```python
from build123d import *

# Parameters (mm, degrees)
SKETCH1_R           = 20.5
BOSS_EXTRUDE1_DEPTH = 2
SKETCH2_R           = 2.675
CUT_EXTRUDE1_DEPTH  = 2
BOSS_EXTRUDE2_START = 0.4
SKETCH3_R           = 3.425
SKETCH3_R_2         = 2.675
BOSS_EXTRUDE2_DEPTH = 0.4
SKETCH4_R           = 2
CUT_EXTRUDE2_DEPTH  = 2


with BuildPart() as part:
    # Sketch1 → Boss-Extrude1 (new body)
    with BuildSketch(Plane(origin=(0, 0, 0), x_dir=(1, 0, 0), z_dir=(0, 1, 0))):
        with Locations(Location((0, 0, 0), (0, 0, 270))):
            Circle(SKETCH1_R)
    extrude(amount=BOSS_EXTRUDE1_DEPTH)

    # Sketch2 → Cut-Extrude1 (cut)
    with BuildSketch(Plane(origin=(0, 2, 0), x_dir=(1, 0, 0), z_dir=(0, 1, 0))):
        with Locations(Location((0, 0, 0), (0, 0, 270))):
            Circle(SKETCH2_R)
    extrude(amount=-CUT_EXTRUDE1_DEPTH, mode=Mode.SUBTRACT)

    # Sketch3 → Boss-Extrude2 (add)
    with BuildSketch(Plane(origin=(0, 2, 0), x_dir=(1, 0, 0), z_dir=(0, 1, 0)).offset(BOSS_EXTRUDE2_START)):
        with Locations(Location((0, 0, 0), (0, 0, 270))):
            Circle(SKETCH3_R)
        with Locations(Location((0, 0, 0), (0, 0, 270))):
            Circle(SKETCH3_R_2, mode=Mode.SUBTRACT)
    extrude(amount=-BOSS_EXTRUDE2_DEPTH)

    # Sketch4 → Cut-Extrude2 (cut)
    with BuildSketch(Plane(origin=(0, 2, 0), x_dir=(1, 0, 0), z_dir=(0, 1, 0))):
        with Locations(Location((0, 16.68859089, 0), (0, 0, 270))):
            Circle(SKETCH4_R)
    extrude(amount=-CUT_EXTRUDE2_DEPTH, mode=Mode.SUBTRACT)


solid = part.part
```
Design review of the part built by this model. Coordinates are the model's own, in mm. A direction names the side the tool comes from. Give positions to 0.01 mm unless a question says otherwise; leave off trailing zeros. Write each loop counter-clockwise with the first axis right and the second up, starting at its lowest first coordinate (ties: lowest second). Pieces come first, ordered by that corner, then holes. Notation, with made-up numbers: (-40, 48) - (19, 48) arc R23 ccw to (19, 75) - close; hole circle Ø7 at (48.25, 59.25). An arc over 180 degrees is marked (long way). Return JSON: item names as keys, results as strings. Group by question number.
(1) Machinability: for faces 1 (the cylindrical face through (1.029, 2.203, 3.267)), 2 (the cylindrical face through (-2.61, 1.22, -0.58)), which of the approach directions +Z, -Z, +X, -X, +Y, -Y give a long, thin tool a straight path to every point of the face, cutting with its end or side? Answer none if there is none.
(2) Mouldability with a two-part tool opening along X and no side actions: class faces 3 (the cylindrical face through (-20.013, 0.986, -4.444)), 4 (the cylindrical face through (-0.766, 1.014, -14.841)), 5 (the flat face through (0, 0, 4)) as +X half, -X half, draft (parallel to the pull), parting line (faces both ways), or undercut.
(3) We need section C-C, the plane y = 1.5. Give the boundary of the cut face in (x, z) (3 decimals), then the cut area to 3 significant figures.
(4) We need section D-D, the plane x = 4.5. Give the boundary of the cut face in (y, z), then the cut area to 3 significant figures.
(5) We need section B-B, the plane z = 0. Give the boundary of the cut face in (x, y) (3 decimals).
(6) To check wall thickness, follow probe 1 along X at (y, z) = (0.8, 0) (3 decimals); probe 2 along Z at (x, y) = (1.5, 0.2); probe 3 along Y at (x, z) = (12.5, -4). State the ranges of each line that lie inside material, in increasing order.
(7) We need section A-A, the plane x = 0. Give the boundary of the cut face in (y, z) (3 decimals), then the cut area to 3 significant figures.
Reported:
{
 "1": {"face 1": "+Y", "face 2": "+Y, -Y"},
 "2": {"face 3": "parting line", "face 4": "undercut", "face 5": "draft"},
 "3": {"outline": "circle Ø41 at (0, 0); hole circle Ø5.35 at (0, 0); hole circle Ø4 at (0, -16.689)", "area": "1,290 mm2"},
 "4": {"outline": "(0, -20) - (2, -20) - (2, 20) - (0, 20) - close", "area": "80.0 mm2"},
 "5": {"outline": "(-20.5, 0) - (-2.675, 0) - (-2.675, 2.4) - (-3.425, 2.4) - (-3.425, 2) - (-20.5, 2) - close; (2.675, 0) - (20.5, 0) - (20.5, 2) - (3.425, 2) - (3.425, 2.4) - (2.675, 2.4) - close"},
 "6": {"probe 1": "x = -20.5 to -2.675, 2.675 to 20.5", "probe 2": "z = -20.45 to -18.01, -15.37 to -2.21, 2.21 to 20.45", "probe 3": "y = 0 to 2"},
 "7": {"outline": "(0, -20.5) - (2, -20.5) - (2, -18.689) - (0, -18.689) - close; (0, -14.689) - (2, -14.689) - (2, -3.425) - (2.4, -3.425) - (2.4, -2.675) - (0, -2.675) - close; (0, 2.675) - (2.4, 2.675) - (2.4, 3.425) - (2, 3.425) - (2, 20.5) - (0, 20.5) - close", "area": "63.9 mm2"}
}
